```python
from build123d import *

# Parameters (mm, degrees)
SKETCH3_W          = 2
SKETCH3_H          = 3
CUT_EXTRUDE1_DEPTH = 32.940413272
CHAMFER1_SIZE      = 0.5


with BuildPart() as part:
    # Sketch2 → Revolve1 (revolve)
    with BuildSketch(Plane.XY):
        with BuildLine():
            Line((0, 0), (0, 31.3))
            ThreePointArc((0, 31.3), (2.015254326, 30.465254326), (2.85, 28.45))
            Line((2.85, 28.45), (2.85, 13.5))
            Line((2.85, 13.5), (4, 13.5))
            Line((4, 13.5), (4.5, 13))
            Line((4.5, 13), (4.5, 10))
            Line((4.5, 10), (3.2, 10))
            Line((3.2, 10), (3.2, 8))
            Line((3.2, 8), (3, 8))
            Line((3, 8), (3, 0))
            Line((3, 0), (0, 0))
        make_face()
    revolve(axis=Axis((0, 0, 0), (0, 1, 0)))

    # Sketch3 → Cut-Extrude1 (cut, symmetric)
    with BuildSketch(Plane.XY):
        with Locations((-4.75, 12.5)):
            Rectangle(SKETCH3_W, SKETCH3_H)
    cut_extrude1 = extrude(amount=CUT_EXTRUDE1_DEPTH, both=True, mode=Mode.SUBTRACT)

    # Mirror1: Cut-Extrude1 across plane
    add(cut_extrude1.mirror(Plane(origin=(0, 0, 0), x_dir=(0, 0, 1), z_dir=(1, 0, 0))), mode=Mode.SUBTRACT)

    # Chamfer1
    chamfer1_edges = [part.edges().sort_by_distance(p)[0] for p in [
        (-3, 0, 0),
    ]]
    chamfer(chamfer1_edges, length=CHAMFER1_SIZE)


solid = part.part
```
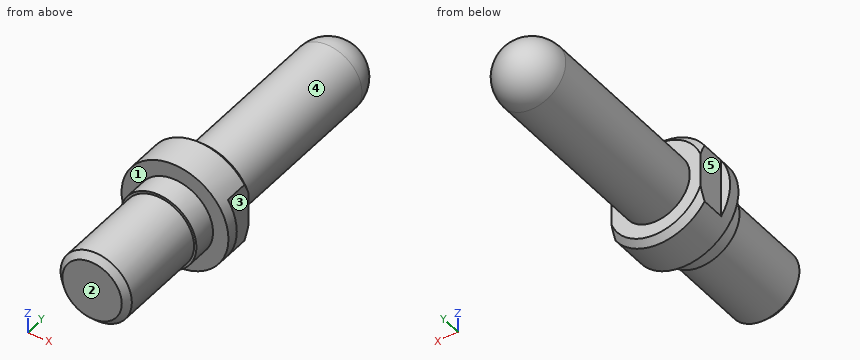
Work out the finished part from the listing and answer in its coordinate system (mm). Face numbers are marked on the shaded views. A direction names the side the tool comes from. Give positions to 0.01 mm unless a question says otherwise; leave off trailing zeros. Loops run counter-clockwise (first coordinate to the right, second up) from the corner with the lowest first, then second, coordinate; pieces in that order, holes last. Notation, with made-up numbers: (63, -20.5) -> (96, -20.5) arc R22 ccw to (96, -6.5) -> close; hole circle Ø9 at (-11, -34). An arc over 180 degrees is marked (long way). Put each result on its own line as item: value. Start each with the question number.
Item 1: The part is cut by section C-C (y = 8.5). Give the vertices of the cut face in (x, z), then the cut area to 3 significant figures.
Item 2: The part is cut by section B-B (z = 0). Give the vertices of the cut face in (x, y), then the cut area to 3 significant figures.
Item 3: Find the intervals of material crossed by L1, parallel to Y at x = 3, z = -1.25; L2, parallel to X at y = 12.5, z = -2; L3, parallel to Z at x = 1.75, y = 24, in increasing order. Write a range as [from, to].
Item 4: The part is cut by section D-D (y = 20.5). Give the vertices of the cut face in (x, z).
Item 5: The part is cut by section A-A (x = 0). Give the vertices of the cut face in (y, z).
Item 6: Each of these flat-tipped pins is pushed along its axis until it touches: P1, Ø2, axis at x = -3, z = -1.5, coming from the +Y side; P2, Ø1, axis at x = 0.5, y = 20, coming from the -Z side; P3, Ø2, axis at x = -0.5, y = 7.5, coming from the -Z side. Where does it stop, or does it pass through?
Item 7: Which of the six approach directions +Z, -Z, +X, -X, +Y, -Y give full straight-line access (tool end or side, diameter ignored) to the marked faces 1, 2, 3, 4 and 5?
Answers below:
1. outline: circle Ø6.4 at (0, 0)
1. area: 32.2 mm2
2. outline: (-4.5, 10) -> (-3.2, 10) -> (-3.2, 8) -> (-3, 8) -> (-3, 0.5) -> (-2.5, 0) -> (2.5, 0) -> (3, 0.5) -> (3, 8) -> (3.2, 8) -> (3.2, 10) -> (4.5, 10) -> (4.5, 11) -> (3.75, 11) -> (3.75, 13.5) -> (2.85, 13.5) -> (2.85, 28.45) arc R2.85 ccw to (-2.85, 28.45) -> (-2.85, 13.5) -> (-3.75, 13.5) -> (-3.75, 11) -> (-4.5, 11) -> close
2. area: 186 mm2
3. L1: [10, 13.5]
3. L2: [-3.75, 3.75]
3. L3: [-2.25, 2.25]
4. outline: circle Ø5.7 at (0, 0)
5. outline: (0, -2.5) -> (0.5, -3) -> (8, -3) -> (8, -3.2) -> (10, -3.2) -> (10, -4.5) -> (13, -4.5) -> (13.5, -4) -> (13.5, -2.85) -> (28.45, -2.85) arc R2.85 ccw to (28.45, 2.85) -> (13.5, 2.85) -> (13.5, 4) -> (13, 4.5) -> (10, 4.5) -> (10, 3.2) -> (8, 3.2) -> (8, 3) -> (0.5, 3) -> (0, 2.5) -> close
6. P1: y = 30.06
6. P2: z = -2.85
6. P3: z = -3.2
7. face 1: -Y
7. face 2: +Z, -Z, +X, -X, -Y
7. face 3: +Z, -Z, +X, +Y
7. face 4: +Y
7. face 5: +Z, -Z, -X, +Y
